Check sheet for the modelled part. Datum: model origin and axes. Units: mm. A direction names the side the tool comes from. Give positions to 0.01 mm unless a question says otherwise; leave off trailing zeros. Order: outer loops, then holes, each group sorted by start corner. A loop starts at its lowest first (then second) coordinate and runs counter-clockwise, first axis right, second up. Notation, with made-up numbers: (-25, 35) -> (14, 35) arc R29 ccw to (14, 68) -> close; hole circle Ø10 at (10, 85.25). An arc over 180 degrees is marked (long way). Answer in a Markdown table with one row per item. Add a question column.
(1) Cross-section at A-A (x = 0). Record the cut outline in (y, z), then the cut area to 3 significant figures.
(2) Cross-section at C-C (x = 4). Record the cut outline in (y, z).
(3) Go/stop test with flat-tipped pins: pin 1 (1 mm diameter, centred on x = -4, z = 5, fed in from -Y); pin 2 (4 mm diameter, centred on x = 2.5, z = 5.5, fed in from -Y); pin 3 (3 mm diameter, centred on x = -2, z = 3.5, fed in from +Y). Record where each tip stops, or that it passes through.
(4) Cross-section at B-B (y = 4). Record the cut outline in (x, z).
(5) Thickness scan on L1, parallel to Y at x = 0, z = 3; L2, parallel to X at y = -3, z = 7.25; L3, parallel to Y at x = -3.75, z = 5. Record the ranges inside material, lowest first. Write a range as [from, to].
(6) Release check for a two-part mould opening along Y. For faces 1 (the face through (3, 0, 7.68)), 2 (the face through (-6.094, -0.268, 3.786)), 3 (the face through (-3, -2, 0.68)) record: released by +Y, released by -Y, zero draft, split by the parting line, or undercut.
(7) Cross-section at D-D (z = 3.5). Record the cut outline in (x, y).
(8) Set-up check for faces 4 (the face through (3, 0, 0)), 5 (the face through (3, -2, 0.68)): record each of +Z, -Z, +X, -X, +Y, -Y from which the full face is reachable in a straight line by a thin tool's end or side.
Autodesk Inventor part; units mm, degrees
ref_plane "YZ Plane" through (0, 0, 0) normal (1, 0, 0) x (0, 1, 0)
ref_plane "XZ Plane" through (0, 0, 0) normal (0, 1, 0) x (-1, 0, 0)
ref_plane "XY Plane" through (0, 0, 0) normal (0, 0, 1) x (1, 0, 0)
sketch "Sketch1" plane through (0, 0, 0) normal (0, 0, 1) x (1, 0, 0)
  circle A0 centre (0, 0) radius 6.1
  dimension "d0" = 12.2
extrude "Extrusion1" add sketch "Sketch1" along normal blind 7.68
sketch "Sketch2" plane through (0, 0, 7.68) normal (0, 0, 1) x (1, 0, 0)
  circle A0 centre (0, 0) radius 6.1
  line L0 (0, 4) -> (0, 0) construction
  line L1 (0, 0) -> (-3.4641, -2) construction
  line L2 (3.4641, -2) -> (0, 0) construction
  dimension "d3" = 120
  dimension "d4" = 120
  dimension "d5" = 4
hole "Hole1" at (0, 4, 7.68) at (-3.4641, -2, 7.68) at (3.4641, -2, 7.68) direction (0, 0, -1) diameter 3 depth 7
sketch "Sketch3" plane through (0, 0, 0) normal (0, 0, -1) x (-1, 0, 0)
  point P0 (0, 0)
hole "Hole2" at (0, 0, 0) direction (0, 0, 1) diameter 4 end through all
equation "\"d4\" = d3"
properties part number "ScissorPin" material "ABS Plastic"
Answer below:
| question | item | result |
|---|---|---|
| 1 | outline | (-6.1, 0) -> (-2, 0) -> (-2, 7.68) -> (-6.1, 7.68) -> close; (2, 0) -> (6.1, 0) -> (6.1, 7.68) -> (5.5, 7.68) -> (5.5, 0.68) -> (2.5, 0.68) -> (2.5, 7.68) -> (2, 7.68) -> close |
| 1 | area | 42.0 mm² |
| 2 | outline | (-4.61, 0) -> (4.61, 0) -> (4.61, 7.68) -> (-0.6, 7.68) -> (-0.6, 0.68) -> (-3.4, 0.68) -> (-3.4, 7.68) -> (-4.61, 7.68) -> close |
| 3 | pin 1 | stops at y = -5 |
| 3 | pin 2 | stops at y = -6.08 |
| 3 | pin 3 | stops at y = 6.08 |
| 4 | outline | (-4.61, 0) -> (4.61, 0) -> (4.61, 7.68) -> (1.5, 7.68) -> (1.5, 0.68) -> (-1.5, 0.68) -> (-1.5, 7.68) -> (-4.61, 7.68) -> close |
| 5 | L1 | y = [-6.1, -2], [2, 2.5], [5.5, 6.1] |
| 5 | L2 | x = [-5.31, -4.58], [-2.35, 2.35], [4.58, 5.31] |
| 5 | L3 | y = [-4.81, -3.47], [-0.53, 4.81] |
| 6 | face 1 | zero draft |
| 6 | face 2 | split by the parting line |
| 6 | face 3 | undercut |
| 7 | outline | circle Ø12.2 at (0, 0); hole circle Ø3 at (-3.46, -2); hole circle Ø4 at (0, 0); hole circle Ø3 at (0, 4); hole circle Ø3 at (3.46, -2) |
| 8 | face 4 | -Z, +X, -X, +Y, -Y |
| 8 | face 5 | +Z |
